Work out the finished part from the listing and answer in its coordinate system (mm). A direction names the side the tool comes from. Round coordinates to 2 decimals unless told otherwise and drop trailing zeros. Order: outer loops, then holes, each group sorted by start corner. A loop starts at its lowest first (then second) coordinate and runs counter-clockwise, first axis right, second up. Notation, with made-up numbers: (-6.75, 78) - (5.25, 78) arc R13 cw to (5.25, 94) - close; hole circle Ø7 at (66, 83.5). An arc over 180 degrees is marked (long way). Put each result on its own line as item: value.
Autodesk Fusion 360 part; units mm, degrees
sketch "스케치1" plane through (0, 0, 0) normal (0, 1, 0) x (1, 0, 0)
  circle A0 centre (0, 0) radius 22.5
  line L0 (0, 0) -> (0, -24)
  line L1 (0, -24) -> (15.2, -24)
  line L2 (15.2, -24) -> (-15.2, -24)
  line L3 (-15.2, -24) -> (-15.2, -49.4)
  line L4 (-15.2, -49.4) -> (15.2, -49.4)
  line L5 (15.2, -49.4) -> (15.2, -24)
  circle A1 centre (0, 0) radius 25
  line L6 (-15.2, -24) -> (-15.2, -18.5)
  line L7 (15.2, -24) -> (15.2, -18.5685)
  line L8 (0, -36.7) -> (0, -34.2)
  line L9 (10.2, -44.4) -> (-10.2, -44.4)
  line L10 (-10.2, -44.4) -> (-10.2, -24)
  line L11 (-10.2, -24) -> (10.2, -24)
  line L12 (10.2, -24) -> (10.2, -44.4)
  line L13 (10.2, -44.4) -> (-10.2, -24) construction
  line L14 (-10.2, -44.4) -> (10.2, -24) construction
  point P0 (0, -36.7)
  point P1 (0, -34.2)
  dimension "d1" = 45
  dimension "d2" = 24
  dimension "d3" = 15.2
  dimension "d4" = 30.4
  dimension "d5" = 25.4
  dimension "d8" = 50
  dimension "d13" = 2.5
  dimension "d14" = 20.4
  dimension "d15" = 20.4
extrude "돌출1" add sketch "스케치1" along normal blind 10 contours L1 L2 A1 L11 | L1 L2 A1 L7 L11 | L2 A1 L6 L11 | L1 L2 L3 L4 L5 L9 L10 L12 picked at (-16.0726, -17.9881)
extrude "돌출2" add sketch "스케치1" against normal blind 10 contours L1 L2 A1 L11 picked at (-16.0726, -17.9881)
sketch "스케치2" plane through (0, 0, 49.4) normal (0, 0, 1) x (-1, 0, 0)
  line L0 (15.2, 0) -> (-15.2, 0)
  line L1 (-15.2, 0) -> (-15.2, -10)
  line L2 (-15.2, -10) -> (15.2, -10)
  line L3 (15.2, -10) -> (15.2, 0)
  circle A0 centre (0, -5) radius 2.6
  dimension "d18" = 5.2
extrude "돌출3" cut sketch "스케치2" against normal blind 11 contours A0
sketch "스케치3" plane through (-10.2, 0, 0) normal (1, 0, 0) x (0, 1, 0)
  line L0 (0, 44.4) -> (0, 24)
  line L1 (0, 24) -> (10, 24)
  line L2 (10, 24) -> (10, 44.4)
  line L3 (10, 44.4) -> (0, 44.4)
  circle A0 centre (5, 34.2) radius 2.6
  dimension "d21" = 5.2
extrude "돌출4" cut sketch "스케치3" along normal blind 33 contours A0
extrude "돌출5" cut sketch "스케치3" against normal blind 17 contours A0
1) A cutting plane is placed at C-C on z = 34.2. Write down the section's boundary in (x, y), then the cut area to 3 significant figures.
Findings below:
outline: (-15.2, 0) - (-10.2, 0) - (-10.2, 2.4) - (-15.2, 2.4) - close; (-15.2, 7.6) - (-10.2, 7.6) - (-10.2, 10) - (-15.2, 10) - close; (10.2, 0) - (15.2, 0) - (15.2, 2.4) - (10.2, 2.4) - close; (10.2, 7.6) - (15.2, 7.6) - (15.2, 10) - (10.2, 10) - close
area: 48.0 mm2
2) For a pull along X with two mould halves and no side action, classify faces 5 (the cylindrical face through (-12.66, 4.44, 31.66)), 6 (the flat face through (0, 0, 24)), 7 (the flat face through (15.2, 5, 38)) as pulls with the +X half, pulls with the -X half, needs draft (parallel to the pull), parting line crosses it, or undercut.
Findings below:
face 5: needs draft
face 6: undercut
face 7: pulls with the +X half
3) A cutting plane is placed at B-B on x = 0. Write down the section's boundary in (y, z).
Findings below:
outline: (-10, -25) - (10, -25) - (10, -22.5) - (-10, -22.5) - close; (-10, 22.5) - (10, 22.5) - (10, 24) - (-10, 24) - close; (0, 44.4) - (2.4, 44.4) - (2.4, 49.4) - (0, 49.4) - close; (7.6, 44.4) - (10, 44.4) - (10, 49.4) - (7.6, 49.4) - close
4) A cutting plane is placed at A-A on y = 5. Write down the section's boundary in (x, z).
Findings below:
outline: (-15.2, 19.85) arc R25 ccw (long way) to (15.2, 19.85) - (15.2, 31.6) - (10.2, 31.6) - (10.2, 24) - (-10.2, 24) - (-10.2, 31.6) - (-15.2, 31.6) - close; (-15.2, 36.8) - (-10.2, 36.8) - (-10.2, 44.4) - (-2.6, 44.4) - (-2.6, 49.4) - (-15.2, 49.4) - close; (2.6, 44.4) - (10.2, 44.4) - (10.2, 36.8) - (15.2, 36.8) - (15.2, 49.4) - (2.6, 49.4) - close; hole circle Ø45 at (0, 0)
5) For faces 1 (the cylindrical face through (-1.2, 7.307, 46.935)), 2 (the flat face through (2, 3, 44.4)), 3 (the flat face through (-15.2, 5, 38)), 4 (the flat face through (-22.3, -10, -4.2)), determine the directions among +Z, -Z, +X, -X, +Y, -Y from which every point of the face is accessible in a straight line to the end or side of a thin tool.
Findings below:
face 1: +Z
face 2: +Y, -Y
face 3: +Z, -X, +Y, -Y
face 4: +Z, -Z, +X, -X, -Y
6) Given pin 1 Ø3 at (y, z) = (1, 13) entering from -X; pin 2 Ø12 at (y, z) = (-3.5, 23) entering from +X; pin 3 Ø6 at (x, y) = (-19.5, -7) entering from +Z, each flat-ended and moving along its own axis, determine where each tip first touches the part or whether it passes through.
Findings below:
pin 1: stops at x = -22.2
pin 2: stops at x = 18.33
pin 3: stops at z = 18.78
7) A cutting plane is placed at D-D on z = 0. Write down the section's boundary in (x, y), then the cut area to 3 significant figures.
Findings below:
outline: (-25, -10) - (-22.5, -10) - (-22.5, 10) - (-25, 10) - close; (22.5, -10) - (25, -10) - (25, 10) - (22.5, 10) - close
area: 100 mm2
8) Straight lines are drawn through the part: L1, parallel to X at y = -3.75, z = 0; L2, parallel to X at y = 5, z = 48; L3, parallel to Z at x = -8, y = 4.5. For each, find the intervals that lie inside material, in ascending order. Write a range as from..to.
Findings below:
L1: x = -25..-22.5, 22.5..25
L2: x = -15.2..-2.6, 2.6..15.2
L3: z = -23.69..-21.03, 21.03..24, 44.4..49.4
